Can you work these out from the drawing? Everything is in mm from the part's minimum corner. Round coordinates to 2 decimals unless told otherwise and drop trailing zeros. Loops run counter-clockwise (first coordinate to the right, second up) from the corner with the lowest first, then second, coordinate; pieces in that order, holes last. Notation, with made-up numbers: (54.5, 28) -> (90.5, 28) arc R21 ccw to (90.5, 54) -> close; hole circle Ø6 at (50, 4). An arc over 180 degrees is marked (long way). One line per item, written item: value.
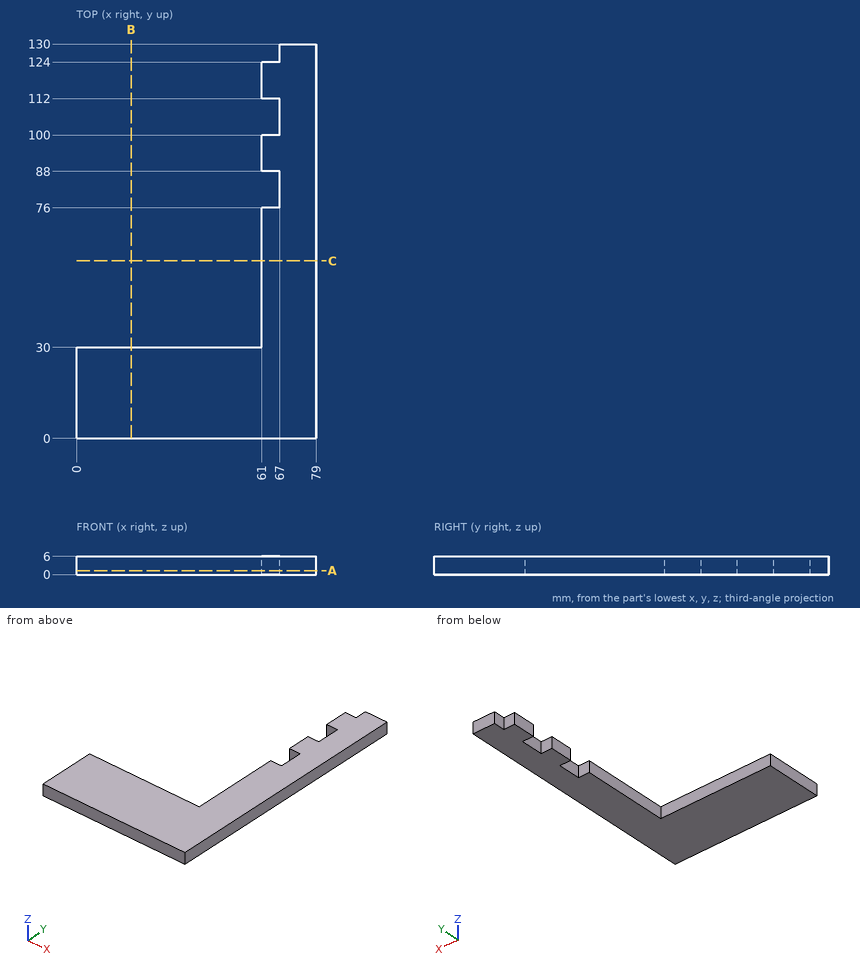
(1) Imagine slicing it at B-B on x = 18. Write out the boundary of the cut face in (y, z), then the cut area to 3 significant figures.
Results below:
outline: (0, 0) -> (30, 0) -> (30, 6) -> (0, 6) -> close
area: 180 mm²
(2) Imagine slicing it at A-A on z = 1.3. Write out the boundary of the cut face in (x, y).
Results below:
outline: (0, 0) -> (79, 0) -> (79, 130) -> (67, 130) -> (67, 124) -> (61, 124) -> (61, 112) -> (67, 112) -> (67, 100) -> (61, 100) -> (61, 88) -> (67, 88) -> (67, 76) -> (61, 76) -> (61, 30) -> (0, 30) -> close
(3) Please list where these lines run through material, in increasing order: L1, parallel to Y at x = 38.5, z = 2.7; L2, parallel to X at y = 96.5, z = 0.35; L3, parallel to X at y = 85.5, z = 2.35.
Results below:
L1: y = 0 to 30
L2: x = 61 to 79
L3: x = 67 to 79
(4) Imagine slicing it at C-C on y = 58.5. Write out the boundary of the cut face in (x, z).
Results below:
outline: (61, 0) -> (79, 0) -> (79, 6) -> (61, 6) -> close
(5) For pin 1 Ø3 at (x, z) = (63.5, 4) entering from +Y; pin 2 Ø3 at (x, z) = (44.5, 4.5) entering from +Y; pin 3 Ø1.8 at (x, z) = (65, 4.5) entering from -Y; pin 4 Ø1.8 at (y, z) = (128.5, 4) entering from -X, each with a flat end and sliding along its axis, tell me the tip position at first contact or that it passes through.
Results below:
pin 1: stops at y = 124
pin 2: stops at y = 30
pin 3: stops at y = 0
pin 4: stops at x = 67
